```python
from build123d import *

# Parameters (mm, degrees)
SKICA1_W                 = 140
SKICA1_H                 = 80
P_IDAT_VYSUNUT_M1_DEPTH  = 8
ODEBRAT_VYSUNUT_M1_REACH = 82
SKICA2_W                 = 8
SKICA2_H                 = 5
ZAOBLIT1_R               = 10
ZAOBLIT3_R               = 2


with BuildPart() as part:
    # Skica1 → Přidat vysunutím1 (new body)
    with BuildSketch(Plane(origin=(0, 0, 0), x_dir=(1, 0, 0), z_dir=(0, 1, 0))):
        with Locations((70, 40)):
            Rectangle(SKICA1_W, SKICA1_H)
    extrude(amount=P_IDAT_VYSUNUT_M1_DEPTH)

    # Skica2 → Odebrat vysunutím1 (cut, up to next)
    with BuildSketch(Plane.XY, mode=Mode.PRIVATE) as odebrat_vysunut_m1_sk1:
        with Locations((70, 5.5)):
            Rectangle(SKICA2_W, SKICA2_H)
    odebrat_vysunut_m1_tool1 = extrude(odebrat_vysunut_m1_sk1.sketch, amount=-ODEBRAT_VYSUNUT_M1_REACH, mode=Mode.PRIVATE) & part.part
    add(odebrat_vysunut_m1_tool1.solids().sort_by_distance((70, 5.5, 0))[0], mode=Mode.SUBTRACT)

    # Zaoblit1
    zaoblit1_edges = [part.edges().sort_by_distance(p)[0] for p in [
        (0, 4, -80),
        (140, 4, -80),
        (140, 4, 0),
        (0, 4, 0),
    ]]
    fillet(zaoblit1_edges, radius=ZAOBLIT1_R)

    # Zaoblit3
    zaoblit3_edges = [part.edges().sort_by_distance(p)[0] for p in [
        (102, 8, 0),
        (38, 8, -80),
        (0, 0, -40),
        (0, 8, -40),
        (70, 0, -80),
        (140, 0, -40),
        (70, 0, 0),
        (2.928932188, 0, -2.928932188),
        (137.071067812, 0, -2.928932188),
        (137.071067812, 0, -77.071067812),
        (2.928932188, 0, -77.071067812),
        (102, 8, -80),
        (38, 8, 0),
        (2.928932188, 8, -2.928932188),
        (2.928932188, 8, -77.071067812),
        (140, 8, -40),
        (137.071067812, 8, -2.928932188),
        (137.071067812, 8, -77.071067812),
    ]]
    fillet(zaoblit3_edges, radius=ZAOBLIT3_R)


solid = part.part
```
Could you check a few things on this model? Use its own coordinates, in mm. A direction names the side the tool comes from. Coordinates: 2 decimals unless noted, no trailing zeros. Write each loop counter-clockwise with the first axis right and the second up, starting at its lowest first coordinate (ties: lowest second). Pieces come first, ordered by that corner, then holes. Notation, with made-up numbers: M 8,30.5 L 59,30.5 A14 cw 59,41.5 Z; hole C 7.5,27 d1. An arc over 180 degrees is marked long. Answer as CSV lines item,"result". Start each with the question number.
1) For faces 1 (the cylindrical face through (2.85, 4.03, -3.01)), 2 (the flat face through (74, 5, -39)), which set-ups out of +Z, -Z, +X, -X, +Y, -Y let a thin tool reach every point of the face, with its end or its side?
2) I want a section at A-A, the plane y = 4.25. Please give me the cut outline in (x, z), and give its area (3 significant figures).
3) For P1, Ø6.5, axis at x = 69.5, z = -32.5, coming from the +Y side; P2, Ø2, axis at x = 74, y = 6.5, coming from the +Z side; P3, Ø1.5, axis at y = 2.5, z = -9, coming from the -X side, each with a flat end and sliding along its axis, tell me the tip position at first contact or that it passes through.
4) Please list where these lines run through material, in increasing order: line 1 (X direction, y = 4, z = -66); line 2 (X direction, y = 1.75, z = -49); line 3 (Z direction, x = 20.5, y = 1.75). Write a range as from..to.
5) We'd pull the mould along X, two halves only. Please class faces 3 (the flat face through (69, 0, -41)), 4 (the flat face through (0, 4, -40)), 5 (the flat face through (66, 5, -39)): +X half, -X half, draft (parallel to the pull), parting line (faces both ways), or undercut.
6) I want a section at B-B, the plane z = -56.5. Please give me the cut outline in (x, y), and give its area (3 significant figures).
Data:
1,face 1,"+Z, -X, +Y, -Y"
1,face 2,"+Z, -Z, +Y"
2,outline,"M 0,-70 A10 ccw 10,-80 L 66,-80 L 66,0 L 10,0 A10 ccw 0,-10 Z; M 74,-80 L 130,-80 A10 ccw 140,-70 L 140,-10 A10 ccw 130,0 L 74,0 Z"
2,area,"10,500 mm^2"
3,P1,"stops at y = 3"
3,P2,"stops at z = 0"
3,P3,"stops at x = 0"
4,line 1,"x = 0..66, 74..140"
4,line 2,"x = 0.02..139.98"
4,line 3,"z = -79.98..-0.02"
5,face 3,"draft"
5,face 4,"-X half"
5,face 5,"undercut"
6,outline,"M 0,2 A2 ccw 2,0 L 138,0 A2 ccw 140,2 L 140,6 A2 ccw 138,8 L 74,8 L 74,3 L 66,3 L 66,8 L 2,8 A2 ccw 0,6 Z"
6,area,"1,080 mm^2"
